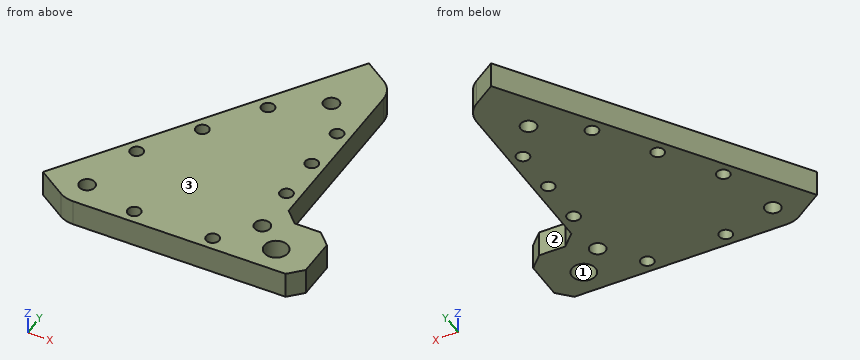
```python
from build123d import *

# Parameters (mm, degrees)
SKETCH_2_R      = 3
SKETCH_2_R_2    = 2.5
SKETCH_2_R_3    = 4.5
EXTRUDE_1_DEPTH = 10


with BuildPart() as part:
    # Эскиз2 → Бобышка-Вытянуть1 (new body)
    with BuildSketch(Plane.XY):
        with BuildLine():
            Line((-34.98035262, -55.873872726), (46.302260596, -55.873872726))
            Line((46.302260596, -55.873872726), (51.302260596, -50.873872726))
            Line((51.302260596, -50.873872726), (51.302260596, -35.873872726))
            Line((51.302260596, -35.873872726), (46.302260596, -30.873872726))
            Line((46.302260596, -30.873872726), (36.302260596, -30.873872726))
            Line((36.302260596, -30.873872726), (31.302260596, -25.873872726))
            Line((31.302260596, -25.873872726), (31.302260596, 41.609691954))
            ThreePointArc((31.302260596, 41.609691954), (30.131736524, 46.304407582), (26.89418963, 49.90006768))
            Line((26.89418963, 49.90006768), (18.037659435, 55.873872726))
            Line((18.037659435, 55.873872726), (-51.302260596, -46.926786271))
            Line((-51.302260596, -46.926786271), (-40.572281655, -54.164248452))
            ThreePointArc((-40.572281655, -54.164248452), (-37.904069667, -55.436920286), (-34.98035262, -55.873872726))
        make_face()
        with Locations((27.302260596, -37.126127274)):
            Circle(SKETCH_2_R, mode=Mode.SUBTRACT)
        with Locations((17.025927685, 31.126127274)):
            Circle(SKETCH_2_R, mode=Mode.SUBTRACT)
        with Locations((-34.98035262, -45.873872726)):
            Circle(SKETCH_2_R, mode=Mode.SUBTRACT)
        with Locations((-28.703706918, -22.364510894)):
            Circle(SKETCH_2_R_2, mode=Mode.SUBTRACT)
        with Locations((-14.723884332, -1.63857158)):
            Circle(SKETCH_2_R_2, mode=Mode.SUBTRACT)
        with Locations((-0.744061745, 19.087367734)):
            Circle(SKETCH_2_R_2, mode=Mode.SUBTRACT)
        with Locations((-14.302260596, -50.873872726)):
            Circle(SKETCH_2_R_2, mode=Mode.SUBTRACT)
        with Locations((15.697739404, -50.873872726)):
            Circle(SKETCH_2_R_2, mode=Mode.SUBTRACT)
        with Locations((26.302260596, 17.873872726)):
            Circle(SKETCH_2_R_2, mode=Mode.SUBTRACT)
        with Locations((26.302260596, -0.126127274)):
            Circle(SKETCH_2_R_2, mode=Mode.SUBTRACT)
        with Locations((26.302260596, -18.126127274)):
            Circle(SKETCH_2_R_2, mode=Mode.SUBTRACT)
        with Locations((37.302260596, -45.873872726)):
            Circle(SKETCH_2_R_3, mode=Mode.SUBTRACT)
    extrude(amount=EXTRUDE_1_DEPTH)


solid = part.part
```
Verification items for the finished model (mm, model axes). Face numbers are marked on the shaded views. Round coordinates to 2 decimals unless told otherwise and drop trailing zeros. Order: outer loops, then holes, each group sorted by start corner. A loop starts at its lowest first (then second) coordinate and runs counter-clockwise, first axis right, second up. Notation, with made-up numbers: (-10, -35.5) -> (41, -35.5) arc R11 ccw to (41, -31.5) -> close; hole circle Ø5 at (-37.75, -28). An arc over 180 degrees is marked (long way). Put each result on its own line as item: value. Start each with the question number.
(1) Section check D-D (y = 8.5). Enter the section's corners in (x, z).
(2) Depth check by flat-ended pin: pin 1 Ø6 at (x, y) = (-0.74, 19.09) entering from -Z; pin 2 Ø4 at (x, y) = (-28.7, -22.36) entering from +Z; pin 3 Ø3 at (y, z) = (34.5, 5) entering from +X; pin 4 Ø3 at (x, z) = (42, 3.5) entering from +Y. Enter the tip coordinate at first touch or a pass-through.
(3) Section check A-A (z = 2). State how many separate pieces and enclosed holes the cut face has, then the cut area to 3 significant figures.
(4) Draft check along Y on the marked faces 1, 2 and 3. Enter one of: +Y half, -Y half, draft (parallel to the pull), parting line (faces both ways), or undercut.
(5) Section check C-C (x = 45). Enter the section's corners in (y, z).
(6) Material ranges on line 1 along X through (y, z) = (-47, 7); line 2 along X through (y, z) = (-46, 1.75); line 3 along Y through (x, z) = (-7.5, 5.25), recorded low to high.
(7) Section check B-B (x = -15.5). Enter the section's corners in (y, z), then the cut area to 3 significant figures.
Completed:
1. outline: (-13.92, 0) -> (31.3, 0) -> (31.3, 10) -> (-13.92, 10) -> close
2. pin 1: stops at z = 0
2. pin 2: passes through
2. pin 3: stops at x = 31.3
2. pin 4: stops at y = -30.87
3. separate pieces: 1
3. enclosed holes: 12
3. area: 5,720 mm2
4. face 1: undercut
4. face 2: +Y half
4. face 3: draft
5. outline: (-55.87, 0) -> (-30.87, 0) -> (-30.87, 10) -> (-55.87, 10) -> close
6. line 1: x = -51.19 to -37.76, -32.2 to 32.95, 41.66 to 51.3
6. line 2: x = -50.68 to -37.98, -31.98 to 32.8, 41.8 to 51.3
6. line 3: y = -55.87 to 18.01
7. outline: (-55.87, 0) -> (-53.07, 0) -> (-53.07, 10) -> (-55.87, 10) -> close; (-48.68, 0) -> (-4.02, 0) -> (-4.02, 10) -> (-48.68, 10) -> close; (0.74, 0) -> (6.15, 0) -> (6.15, 10) -> (0.74, 10) -> close
7. area: 529 mm2
